```python
from build123d import *

# Parameters (mm, degrees)
F0_R     = 4
F1_DEPTH = 10


with BuildPart() as f1:
    # F0 (on Top) → F1 (new body)
    with BuildSketch(Plane.XY):
        with BuildLine():
            ThreePointArc((4.5, -2.1794494718), (4.8733971724, -1.1180339887), (5, 0))
            ThreePointArc((5, 0), (4.8733971724, 1.1180339887), (4.5, 2.1794494718))
            ThreePointArc((4.5, 2.1794494718), (4.1266028276, 1.1180339887), (4, 0))
            ThreePointArc((4, 0), (4.1266028276, -1.1180339887), (4.5, -2.1794494718))
        make_face()
        with BuildLine():
            ThreePointArc((4.5, 2.1794494718), (4.8733971724, 1.1180339887), (5, 0))
            ThreePointArc((5, 0), (4.8733971724, -1.1180339887), (4.5, -2.1794494718))
            ThreePointArc((4.5, -2.1794494718), (10.1180339887, -4.8733971724), (14, 0))
            ThreePointArc((14, 0), (10.1180339887, 4.8733971724), (4.5, 2.1794494718))
        make_face()
        with BuildLine():
            ThreePointArc((13, 0), (9, -4), (5, 0))
            ThreePointArc((5, 0), (9, 4), (13, 0))
        make_face(mode=Mode.SUBTRACT)
        with BuildLine():
            ThreePointArc((4, 0), (4.1266028276, 1.1180339887), (4.5, 2.1794494718))
            ThreePointArc((4.5, 2.1794494718), (-5, 0), (4.5, -2.1794494718))
            ThreePointArc((4.5, -2.1794494718), (4.1266028276, -1.1180339887), (4, 0))
        make_face()
        Circle(F0_R, mode=Mode.SUBTRACT)
    extrude(amount=F1_DEPTH)


solid = f1.part
```
Source: CAD feature listing. Evaluate the final solid. Frame: model axes, mm. Give positions to 0.01 mm unless a question says otherwise; leave off trailing zeros. Order: outer loops, then holes, each group sorted by start corner. A loop starts at its lowest first (then second) coordinate and runs counter-clockwise, first axis right, second up. Notation, with made-up numbers: (6, 53.25) -> (41, 53.25) arc R15 ccw to (41, 74.25) -> close; hole circle Ø1 at (85, 85.25). An arc over 180 degrees is marked (long way). Use a Markdown table: item, result.
Q1. Section A-A (x = 0). Return the cut outline in (y, z).
A:
| item | result |
|---|---|
| outline | (-5, 0) -> (-4, 0) -> (-4, 10) -> (-5, 10) -> close; (4, 0) -> (5, 0) -> (5, 10) -> (4, 10) -> close |
Q2. Pull-direction query (X, two-part tool) for faces 1 (the face through (4.5, 0.4, 0)), 2 (the face through (12.2, -2.4, 4.9)); classes: +X half, -X half, draft (parallel to the pull), parting line (faces both ways), or undercut.
A:
| item | result |
|---|---|
| face 1 | draft |
| face 2 | undercut |
Q3. Section B-B (y = 0.5). Return the cut outline in (x, z), and give its area (3 significant figures).
A:
| item | result |
|---|---|
| outline | (-4.97, 0) -> (-3.97, 0) -> (-3.97, 10) -> (-4.97, 10) -> close; (3.97, 0) -> (5.03, 0) -> (5.03, 10) -> (3.97, 10) -> close; (12.97, 0) -> (13.97, 0) -> (13.97, 10) -> (12.97, 10) -> close |
| area | 30.8 mm^2 |
Q4. First-contact query: P1, Ø5, axis at x = 9, y = 0, coming from the -Z side; P2, Ø2, axis at y = 3, z = 1, coming from the -X side; P3, Ø6, axis at y = -3.5, z = 4.5, coming from the +X side; P4, Ø3, axis at x = 7, z = 4, coming from the +Y side. Flat tips, straight axial feed; report the tip coordinate or a pass-through.
A:
| item | result |
|---|---|
| P1 | through |
| P2 | x = -4.58 |
| P3 | x = 13.97 |
| P4 | y = 4.97 |
Q5. Section D-D (z = 7.75). Return the cut outline in (x, y).
A:
| item | result |
|---|---|
| outline | (4.5, -2.18) arc R5 ccw (long way) to (4.5, 2.18) arc R5 ccw (long way) to start; hole circle Ø8 at (0, 0); hole circle Ø8 at (9, 0) |
Q6. Material intervals for line 1 (X direction, y = -2.75, z = 8); line 2 (X direction, y = -1.75, z = 7); line 3 (X direction, y = -0.75, z = 5.5), sorted ascending. Write a range as [from, to].
A:
| item | result |
|---|---|
| line 1 | [-4.18, -2.9], [2.9, 4.18], [4.82, 6.1], [11.9, 13.18] |
| line 2 | [-4.68, -3.6], [3.6, 5.4], [12.6, 13.68] |
| line 3 | [-4.94, -3.93], [3.93, 5.07], [12.93, 13.94] |
Q7. Section C-C (y = 4.5). Return the cut outline in (x, z), and give its area (3 significant figures).
A:
| item | result |
|---|---|
| outline | (-2.18, 0) -> (2.18, 0) -> (2.18, 10) -> (-2.18, 10) -> close; (6.82, 0) -> (11.18, 0) -> (11.18, 10) -> (6.82, 10) -> close |
| area | 87.2 mm^2 |
